Can you work these out from the model? Positions are in its coordinate system, mm. A direction names the side the tool comes from. Give positions to 0.01 mm unless a question says otherwise; leave off trailing zeros. Loops run counter-clockwise (first coordinate to the right, second up) from the corner with the lowest first, then second, coordinate; pieces in that order, holes last.
from build123d import *

# Parameters (mm, degrees)
BOSS_EXTRUDE1_DEPTH     = 10
CUT_EXTRUDE1_DEPTH      = 25
CUT_EXTRUDE1_DEPTH_BACK = 1.25
SKETCH2_R               = 1.5
CUT_EXTRUDE2_START      = -20
SKETCH6_R               = 1.5
CUT_EXTRUDE2_DEPTH      = 20


with BuildPart() as part:
    # Sketch1 → Boss-Extrude1 (new body)
    with BuildSketch(Plane(origin=(0, 0, 0), x_dir=(0, 0, -1), z_dir=(1, 0, 0))):
        with BuildLine():
            ThreePointArc((-5.664542326, -1.981567074), (-5.004712273, 0.813517905), (-3.164542326, 3.018432939))
            Line((-3.164542326, 3.018432939), (-3.164542326, 2.968432939))
            Line((-3.164542326, 2.968432939), (3.835457674, 2.968432939))
            Line((3.835457674, 2.968432939), (3.835457674, 3.018432939))
            ThreePointArc((3.835457674, 3.018432939), (5.675627611, 0.813517924), (6.335457674, -1.981567032))
            Line((6.335457674, -1.981567032), (6.335457674, -6.981567061))
            Line((6.335457674, -6.981567061), (14.335457674, -6.981567061))
            Line((14.335457674, -6.981567061), (14.335457674, -4.581567061))
            Line((14.335457674, -4.581567061), (8.585457674, -4.581567061))
            Line((8.585457674, -4.581567061), (8.585457674, 2.018432939))
            ThreePointArc((8.585457674, 2.018432939), (7.853224626, 3.786199892), (6.085457674, 4.518432939))
            Line((6.085457674, 4.518432939), (-5.414542326, 4.518432939))
            ThreePointArc((-5.414542326, 4.518432939), (-7.182309279, 3.786199892), (-7.914542326, 2.018432939))
            Line((-7.914542326, 2.018432939), (-7.914542326, -4.581567061))
            Line((-7.914542326, -4.581567061), (-13.664542326, -4.581567061))
            Line((-13.664542326, -4.581567061), (-13.664542326, -6.981567061))
            Line((-13.664542326, -6.981567061), (-5.664542326, -6.981567061))
            Line((-5.664542326, -6.981567061), (-5.664542326, -1.981567074))
        make_face()
    extrude(amount=BOSS_EXTRUDE1_DEPTH)

    # Sketch2 → Cut-Extrude1 (cut, two sides: drawn at the far end of the back side and taken through both)
    # profile 1 of 2: a face of its own
    with BuildSketch(Plane(origin=(0, -4.581567061, 0), x_dir=(1, 0, 0), z_dir=(0, 1, 0)).offset(-CUT_EXTRUDE1_DEPTH_BACK)):
        Polygon((8.233161507, 10.335457674), (6.616580754, 13.135457674), (3.383419246, 13.135457674), (1.766838493, 10.335457674), (3.383419246, 7.535457674), (6.616580754, 7.535457674), align=None)
        with Locations(Location((5, 10.335457674, 0), (0, 0, 270))):
            Circle(SKETCH2_R, mode=Mode.SUBTRACT)
    # profile 2 of 2: a face of its own
    with BuildSketch(Plane(origin=(0, -4.581567061, 0), x_dir=(1, 0, 0), z_dir=(0, 1, 0)).offset(-CUT_EXTRUDE1_DEPTH_BACK)):
        Polygon((8.233161507, -9.664542326), (6.616580754, -6.864542326), (3.383419246, -6.864542326), (1.766838493, -9.664542326), (3.383419246, -12.464542326), (6.616580754, -12.464542326), align=None)
        with Locations(Location((5, -9.664542326, 0), (0, 0, 180))):
            Circle(SKETCH2_R, mode=Mode.SUBTRACT)
    extrude(amount=CUT_EXTRUDE1_DEPTH + CUT_EXTRUDE1_DEPTH_BACK, mode=Mode.SUBTRACT)

    # Sketch6 → Cut-Extrude2 (cut)
    with BuildSketch(Plane(origin=(0, -4.581567061, 0), x_dir=(1, 0, 0), z_dir=(0, 1, 0)).offset(CUT_EXTRUDE2_START)):
        with BuildLine():
            Line((2.410452351, 14.335457674), (0, 14.335457674))
            Line((0, 14.335457674), (0, 12.338937423))
            ThreePointArc((0, 12.338937423), (0.854129864, 13.761085526), (2.410452351, 14.335457674))
        make_face()
        with BuildLine():
            Line((10, 14.335457674), (7.589547649, 14.335457674))
            ThreePointArc((7.589547649, 14.335457674), (9.145870136, 13.761085526), (10, 12.338937423))
            Line((10, 12.338937423), (10, 14.335457674))
        make_face()
        with BuildLine():
            ThreePointArc((2.410452351, -13.664542326), (0.854129864, -13.090170179), (0, -11.668022076))
            Line((0, -11.668022076), (0, -13.664542326))
            Line((0, -13.664542326), (2.410452351, -13.664542326))
        make_face()
        with BuildLine():
            Line((10, -13.664542326), (10, -11.668022076))
            ThreePointArc((10, -11.668022076), (9.145870136, -13.090170179), (7.589547649, -13.664542326))
            Line((7.589547649, -13.664542326), (10, -13.664542326))
        make_face()
        with Locations(Location((5, 10.335457674, 0), (0, 0, 270))):
            Circle(SKETCH6_R)
        with Locations(Location((5, -9.664542326, 0), (0, 0, 180))):
            Circle(SKETCH6_R)
    extrude(amount=CUT_EXTRUDE2_DEPTH, mode=Mode.SUBTRACT)


solid = part.part
(1) Suppose I cut it at D-D on z = -8.25. List the corners of the cut face in (x, y) for me, plus the area to 3 significant figures.
Returned:
outline: (0, -6.98) - (10, -6.98) - (10, 3.27) - (7.03, 3.27) - (7.03, -5.83) - (2.97, -5.83) - (2.97, 3.27) - (0, 3.27) - close
area: 65.6 mm2
(2) Which directions (+Z, -Z, +X, -X, +Y, -Y) give clear straight access to the entire face, cutting with the end or side of a thin tool? Please do faces 5 (the flat face through (5, -4.582, 13)), 6 (the flat face through (5, 4.518, 0)), 7 (the flat face through (7.05, -2.06, -8.29)), 8 (the flat face through (5, 2.968, 0)), 9 (the flat face through (10, 3.5, -1.2)).
Returned:
face 5: +Z, +X, -X, +Y
face 6: +Z, -Z, +X, -X, +Y
face 7: +Y
face 8: +X, -X, -Y
face 9: +Z, -Z, +X, +Y, -Y
(3) Please list where these lines run through material, in increasing order: probe 1 along Z at (x, y) = (5, -6.35); probe 2 along Z at (x, y) = (7, -6); probe 3 along Z at (x, y) = (6, -0.25).
Returned:
probe 1: z = -14.34 to -11.84, -8.84 to -6.34, 5.66 to 8.16, 11.16 to 13.66
probe 2: z = -14.34 to -6.34, 5.66 to 13.66
probe 3: z = -7.54 to -6.09, 5.42 to 6.86
(4) Thinking about a two-plate mould opening in Z: for faces 1 (the cylindrical face through (4.93, 4.296, 6.446)), 2 (the flat face through (0, 3.5, -1.2)), 3 (the flat face through (2.56, -5.22, 11.04)), 4 (the flat face through (6, -5.832, 8)), which applies, pulls with the +Z half, pulls with the -Z half, needs draft (parallel to the pull), parting line crosses it, or undercut?
Returned:
face 1: pulls with the +Z half
face 2: needs draft
face 3: undercut
face 4: undercut
(5) Suppose I cut it at C-C on y = -0.5. List the corners of the cut face in (x, z) for me, plus the area to 3 significant figures.
Returned:
outline: (0, -8.59) - (2.78, -8.59) - (3.38, -7.54) - (6.62, -7.54) - (7.22, -8.59) - (10, -8.59) - (10, -6.16) - (0, -6.16) - close; (0, 5.49) - (10, 5.49) - (10, 7.91) - (7.22, 7.91) - (6.62, 6.86) - (3.38, 6.86) - (2.78, 7.91) - (0, 7.91) - close
area: 40.5 mm2
(6) Suppose I cut it at A-A on z = 10. List the corners of the cut face in (x, y) for me.
Returned:
outline: (0, -6.98) - (3.54, -6.98) - (3.54, -5.83) - (1.96, -5.83) - (1.96, -4.58) - (0, -4.58) - close; (6.46, -6.98) - (10, -6.98) - (10, -4.58) - (8.04, -4.58) - (8.04, -5.83) - (6.46, -5.83) - close
(7) Suppose I cut it at B-B on x = 5. Give the number of separate pieces and of enclosed holes in the cut face, plus the area to 3 significant figures.
Returned:
separate pieces: 3
enclosed holes: 0
area: 64.8 mm2
(8) Will these pins go through, and if not, where does the flat tip stop? P1, Ø6, axis at y = 3, z = -10.5, coming from the +X side; P2, Ø4.5, axis at x = 4, z = -12.5, coming from the +Y side; P3, Ø2, axis at x = 8.5, y = 0.5, coming from the +Z side; P4, Ø3.5, axis at x = 4, y = -1.5, coming from the -Z side.
Returned:
P1: stops at x = 10
P2: stops at y = -4.58
P3: stops at z = 7.91
P4: stops at z = -8.59
